The model under review builds one solid part; all positions refer to its coordinate system, in mm. Face numbers are marked on the shaded views. A direction names the side the tool comes from. Give positions to 0.01 mm unless a question says otherwise; leave off trailing zeros. Write each loop counter-clockwise with the first axis right and the second up, starting at its lowest first coordinate (ties: lowest second). Pieces come first, ordered by that corner, then holes. Notation, with made-up numbers: (30.25, -27) - (52.25, -27) arc R31 cw to (52.25, 3) - close; hole circle Ø3 at (-8.5, -25). An arc over 180 degrees is marked (long way). Write item = value, one per line.
```python
from build123d import *

# Parameters (mm, degrees)
SKETCH1_W                    = 34
SKETCH1_H                    = 53
BOSS_EXTRUDE1_DEPTH          = 2
SKETCH2_W                    = 34
SKETCH2_H                    = 2
BOSS_EXTRUDE2_DEPTH          = 27
SKETCH3_W                    = 34
SKETCH3_H                    = 15
BOSS_EXTRUDE3_DEPTH          = 30
SKETCH4_R                    = 9.5
CUT_EXTRUDE1_DEPTH           = 71.632853546
F_94_0_0071_DIAMETER_HOLE1_D = 2.000000064


with BuildPart() as part:
    # Sketch1 → Boss-Extrude1 (new body)
    with BuildSketch(Plane.XY):
        with Locations((17, 26.5)):
            Rectangle(SKETCH1_W, SKETCH1_H)
    extrude(amount=BOSS_EXTRUDE1_DEPTH)

    # Sketch2 → Boss-Extrude2 (add)
    with BuildSketch(Plane.XY.offset(2)):
        with Locations((17, 1)):
            Rectangle(SKETCH2_W, SKETCH2_H)
    extrude(amount=BOSS_EXTRUDE2_DEPTH)

    # Sketch3 → Boss-Extrude3 (add)
    with BuildSketch(Plane(origin=(0, 0, 0), x_dir=(-1, 0, 0), z_dir=(0, 0, -1))):
        with Locations((-17, 7.5)):
            Rectangle(SKETCH3_W, SKETCH3_H)
    extrude(amount=BOSS_EXTRUDE3_DEPTH)

    # Sketch4 → Cut-Extrude1 (cut, through all)
    with BuildSketch(Plane.XY.offset(2)):
        with Locations((17, 34)):
            Circle(SKETCH4_R)
    extrude(amount=-CUT_EXTRUDE1_DEPTH, mode=Mode.SUBTRACT)

    # #94 (0.0071) Diameter Hole1 (through all)
    with Locations(Plane(origin=(0, 0, 0), x_dir=(-1, 0, 0), z_dir=(0, -1, 0))):
        with Locations((-17, -17.304753764), (-17, 15.945587516)):
            Hole(F_94_0_0071_DIAMETER_HOLE1_D / 2)


solid = part.part
```
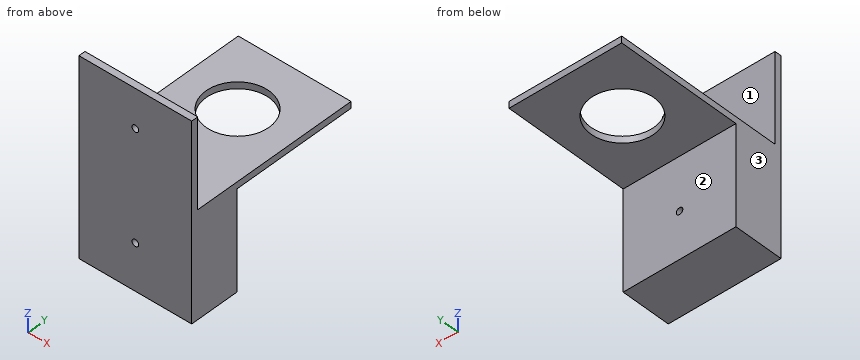
1. Take a section at D-D on x = 13. Give the boundary of the cut face in (y, z).
Findings below:
outline = (0, -30) - (15, -30) - (15, 0) - (25.38, 0) - (25.38, 2) - (2, 2) - (2, 29) - (0, 29) - close; (42.62, 0) - (53, 0) - (53, 2) - (42.62, 2) - close
2. Machinability: for the marked faces 1, 2 and 3, which of the approach directions +Z, -Z, +X, -X, +Y, -Y give a long, thin tool a straight path to every point of the face, cutting with its end or side? Answer none if there is none.
Findings below:
face_1 = +Z, +X, -X, +Y
face_2 = -Z, +X, -X, +Y
face_3 = +Z, -Z, -X, +Y, -Y
3. Take a section at C-C on x = 6. Give the boundary of the cut face in (y, z).
Findings below:
outline = (0, -30) - (15, -30) - (15, 0) - (53, 0) - (53, 2) - (2, 2) - (2, 29) - (0, 29) - close
4. Take a section at A-A on x = 17. Give the boundary of the cut face in (y, z), and give its area (3 significant figures).
Findings below:
outline = (0, -30) - (15, -30) - (15, -16.95) - (0, -16.95) - close; (0, -14.95) - (15, -14.95) - (15, 0) - (24.5, 0) - (24.5, 2) - (2, 2) - (2, 16.3) - (0, 16.3) - close; (0, 18.3) - (2, 18.3) - (2, 29) - (0, 29) - close; (43.5, 0) - (53, 0) - (53, 2) - (43.5, 2) - close
area = 538 mm²
5. Take a section at B-B on y = 34. Give the boundary of the cut face in (x, z), and give its area (3 significant figures).
Findings below:
outline = (0, 0) - (7.5, 0) - (7.5, 2) - (0, 2) - close; (26.5, 0) - (34, 0) - (34, 2) - (26.5, 2) - close
area = 30.0 mm²
6. Insertion check: P1, Ø2, axis at x = 6, z = 9.5, coming from the +Y side; P2, Ø8, axis at x = 25, z = -18, coming from the +Y side; P3, Ø12, axis at x = 22.5, y = 42, coming from the +Z side. Each pin has a flat end and moves straight along its axis. Give the tip position at first contact, or say it passes through.
Findings below:
P1 = 2
P2 = 15
P3 = 2
7. For line 1 (Z direction, x = 17, y = 0.5); line 2 (Z direction, x = 17, y = 5); line 3 (Y direction, x = 17, z = 1.3), list the stretches that pass through material, from the lowest coordinate up. Write a range as from..to.
Findings below:
line_1 = -30..-16.95, -14.95..16.3, 18.3..29
line_2 = -30..-16.95, -14.95..2
line_3 = 0..24.5, 43.5..53
